Geometry check sheet. Reference: the model listing, model coordinates, mm. Coordinates: 2 decimals unless noted, no trailing zeros. Write each loop counter-clockwise with the first axis right and the second up, starting at its lowest first coordinate (ties: lowest second). Pieces come first, ordered by that corner, then holes. Notation, with made-up numbers: (-17.5, 16) - (-12.5, 16) arc R12 ccw to (-12.5, 20) - close; hole circle Ø11 at (37, 17). An arc over 180 degrees is marked (long way). Answer as a JSON object with one key per item and string values. Group by question number.
from build123d import *

# Parameters (mm, degrees)
PAD_DEPTH       = 100
POCKET_DEPTH    = 3
POCKET001_DEPTH = 3


with BuildPart() as part:
    # Sketch → Pad (new body)
    with BuildSketch(Plane.XZ):
        with BuildLine():
            Line((0, 0), (0, 5))
            Line((0, 5), (10, 5))
            ThreePointArc((14.999978, 0), (13.535519, 3.535526), (10, 5))
            Line((0, 0), (14.999978, 0))
        make_face()
    extrude(amount=PAD_DEPTH)

    # Sketch001 → Pocket (cut)
    with BuildSketch(Plane.XY.offset(5)):
        with BuildLine():
            ThreePointArc((8, -10), (5, -7), (2, -10))
            Line((2, -10), (2, -90))
            ThreePointArc((2, -90), (5, -93), (8, -90))
            Line((8, -10), (8, -90))
        make_face()
    extrude(amount=-POCKET_DEPTH, mode=Mode.SUBTRACT)

    # Sketch002 → Pocket001 (cut)
    with BuildSketch(Plane.XY.offset(2)):
        with BuildLine():
            Line((6.7, -10), (6.7, -90))
            ThreePointArc((3.3, -90), (5, -91.7), (6.7, -90))
            Line((3.3, -90), (3.3, -10))
            ThreePointArc((6.7, -10), (5, -8.3), (3.3, -10))
        make_face()
    extrude(amount=-POCKET001_DEPTH, mode=Mode.SUBTRACT)


solid = part.part
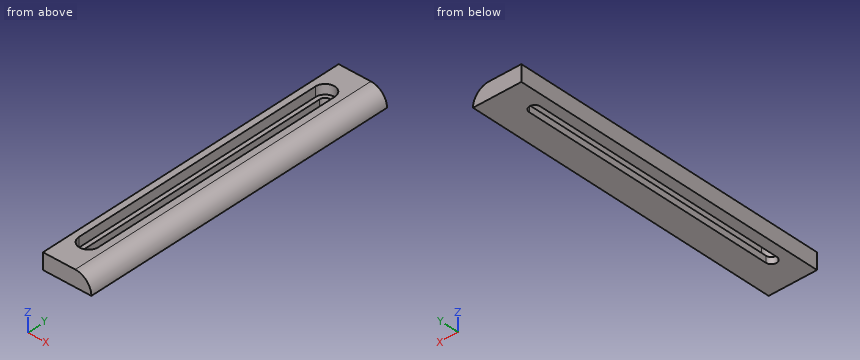
(1) Section check A-A (x = 5). Record the cut outline in (y, z), and give its area (3 significant figures).
(2) Section check C-C (x = 11). Record the cut outline in (y, z), and give its area (3 significant figures).
(3) Section check B-B (y = -26.5). Record the cut outline in (x, z), and give its area (3 significant figures).
(4) Gauge pin test, flat end, axial feed: pin 1 (2.5 mm diameter, centred on y = -44.5, z = 4, fed in from +X). Record the tip position at first contact, or that the pin passes through.
(5) Material ranges on L1, parallel to X at y = -26, z = 0.45; L2, parallel to X at y = -91, z = 2.15; L3, parallel to Y at x = 7.25, z = 4.2, recorded low to high. Write a range as [from, to].
Conclusion:
{
 "1": {"outline": "(-100, 0) - (-91.7, 0) - (-91.7, 2) - (-93, 2) - (-93, 5) - (-100, 5) - close; (-8.3, 0) - (0, 0) - (0, 5) - (-7, 5) - (-7, 2) - (-8.3, 2) - close", "area": "75.2 mm^2"},
 "2": {"outline": "(-100, 0) - (0, 0) - (0, 4.9) - (-100, 4.9) - close", "area": "490 mm^2"},
 "3": {"outline": "(0, 0) - (3.3, 0) - (3.3, 2) - (2, 2) - (2, 5) - (0, 5) - close; (6.7, 0) - (15, 0) arc R5 ccw to (10, 5) - (8, 5) - (8, 2) - (6.7, 2) - close", "area": "44.8 mm^2"},
 "4": {"pin 1": "stops at x = 14.18"},
 "5": {"L1": "x = [0, 3.3], [6.7, 14.98]", "L2": "x = [0, 2.17], [7.83, 14.51]", "L3": "y = [-100, -91.98], [-8.02, 0]"}
}
